Autodesk Inventor part; units mm, degrees
ref_plane "YZ Plane" through (0, 0, 0) normal (1, 0, 0) x (0, 1, 0)
ref_plane "XZ Plane" through (0, 0, 0) normal (0, 1, 0) x (-1, 0, 0)
ref_plane "XY Plane" through (0, 0, 0) normal (0, 0, 1) x (1, 0, 0)
sketch "Sketch1" plane through (0, 0, 0) normal (1, 0, 0) x (0, 1, 0)
  line L0 (44.6473, -162.2528) -> (44.6473, 101.2722)
  line L1 (-18.8527, 107.6222) -> (-3.6127, 107.6222)
  line L2 (-3.6127, 107.6222) -> (-3.6127, 101.2722)
  line L3 (-18.8527, 101.0377) -> (-18.8527, 107.6222)
  line L4 (2.7373, 107.6222) -> (17.9773, 107.6222)
  line L5 (17.9773, 107.6222) -> (17.9773, 101.2722)
  line L6 (2.7373, 101.2722) -> (2.7373, 107.6222)
  line L7 (24.3273, 107.6222) -> (39.5673, 107.6222)
  line L8 (39.5673, 107.6222) -> (39.5673, 101.2722)
  line L9 (24.3273, 101.2722) -> (24.3273, 107.6222)
  line L10 (39.5673, 101.2722) -> (44.6473, 101.2722)
  line L11 (24.3273, 101.2722) -> (17.9773, 101.2722)
  line L12 (2.7373, 101.2722) -> (-3.6127, 101.2722)
  line L13 (44.6473, -30.4903) -> (-18.8527, -30.4903) construction
  line L14 (-3.6127, -168.6028) -> (-3.6127, -162.2528)
  line L15 (17.9773, -168.6028) -> (17.9773, -162.2528)
  line L16 (2.7373, -162.2528) -> (2.7373, -168.6028)
  line L17 (39.5673, -168.6028) -> (39.5673, -162.2528)
  line L18 (24.3273, -162.2528) -> (24.3273, -168.6028)
  line L19 (39.5673, -162.2528) -> (44.6473, -162.2528)
  line L20 (24.3273, -162.2528) -> (17.9773, -162.2528)
  line L21 (2.7373, -162.2528) -> (-3.6127, -162.2528)
  line L22 (24.3273, -168.6028) -> (39.5673, -168.6028)
  line L23 (-18.8527, -168.6028) -> (-3.6127, -168.6028)
  line L24 (2.7373, -168.6028) -> (17.9773, -168.6028)
  line L25 (-3.6127, 107.6222) -> (-18.8527, 107.6222)
  line L26 (39.5673, 107.6222) -> (24.3273, 107.6222)
  line L27 (17.9773, 107.6222) -> (2.7373, 107.6222)
  line L28 (-18.8527, -20.9653) -> (-12.5027, -20.9653)
  line L29 (-12.5027, -20.9653) -> (-12.5027, 4.4347)
  line L30 (-12.5027, 4.4347) -> (-18.8527, 4.4347)
  line L31 (-18.8527, 23.4847) -> (-12.5027, 23.4847)
  line L32 (-12.5027, 23.4847) -> (-12.5027, 48.8847)
  line L33 (-12.5027, 48.8847) -> (-18.8527, 48.8847)
  line L34 (-18.8527, 67.9347) -> (-12.5027, 67.9347)
  line L35 (-12.5027, 67.9347) -> (-12.5027, 93.3347)
  line L36 (-12.5027, 93.3347) -> (-18.8527, 93.3347)
  line L37 (-3.6127, -168.6028) -> (-3.6127, -162.2528)
  line L38 (2.7373, -162.2528) -> (-3.6127, -162.2528)
  line L39 (-18.8527, -40.0153) -> (-12.5027, -40.0153)
  line L40 (-12.5027, -40.0153) -> (-12.5027, -65.4153)
  line L41 (-12.5027, -65.4153) -> (-18.8527, -65.4153)
  line L42 (-18.8527, -84.4653) -> (-12.5027, -84.4653)
  line L43 (-12.5027, -84.4653) -> (-12.5027, -109.8653)
  line L44 (-12.5027, -109.8653) -> (-18.8527, -109.8653)
  line L45 (-18.8527, -128.9153) -> (-12.5027, -128.9153)
  line L46 (-12.5027, -128.9153) -> (-12.5027, -154.3153)
  line L47 (-12.5027, -154.3153) -> (-18.8527, -154.3153)
  line L48 (-18.8527, 107.6222) -> (-18.8527, 93.3347)
  line L49 (-18.8527, 67.9347) -> (-18.8527, 48.8847)
  line L50 (-18.8527, 23.4847) -> (-18.8527, 4.4347)
  line L51 (-18.8527, -20.9653) -> (-18.8527, -40.0153)
  line L52 (-18.8527, -65.4153) -> (-18.8527, -84.4653)
  line L53 (-18.8527, -109.8653) -> (-18.8527, -128.9153)
  line L54 (-18.8527, -154.3153) -> (-18.8527, -168.6028)
  point P0 (0, 0)
  dimension "d2" = 15.24
  dimension "d3" = 6.35
  dimension "d4" = 15.24
  dimension "d5" = 6.35
  dimension "d7" = 15.24
  dimension "d8" = 9.525
  dimension "d9" = 19.05
  dimension "d10" = 19.05
  dimension "d12" = 25.4
  dimension "d13" = 25.4
  dimension "d14" = 25.4
  dimension "d16" = 6.35
  dimension "d17" = 6.35
  dimension "d20" = 276.225
extrude "Extrusion1" add sketch "Sketch1" along normal blind 6.35
equation "\"d10\" = d9"
equation "\"d13\" = d12"
equation "\"d14\" = d12"
properties part number "Front_Back" material "UHMW, White"
Part model, mm, in its own coordinate system. A direction names the side the tool comes from. Coordinates: 2 decimals unless noted, no trailing zeros. Write each loop counter-clockwise with the first axis right and the second up, starting at its lowest first coordinate (ties: lowest second). Pieces come first, ordered by that corner, then holes. Notation, with made-up numbers: (14.5, 59.25) - (34.5, 59.25) arc R18 cw to (34.5, 82.25) - close; hole circle Ø9 at (-13.5, 70). An arc over 180 degrees is marked (long way). Put each result on its own line as item: value.
1. Band-saw the part on A-A (y = -1). Write the cut outline in (x, z).
Final values:
outline: (0, -162.25) - (6.35, -162.25) - (6.35, 101.27) - (0, 101.27) - close
2. Probe line 1 along Z through (x, y) = (4.25, 22.5); line 2 along Y through (x, z) = (5.5, 0.5). List the from-to ranges inside material, lowest first. Write a range as [from, to].
Final values:
line 1: z = [-162.25, 101.27]
line 2: y = [-12.5, 44.65]
3. Flat gauge pins, fed straight in: pin 1 Ø2 at (x, z) = (5, 78.5) entering from -Y; pin 2 Ø3 at (x, z) = (4.5, -167) entering from +Y; pin 3 Ø1.5 at (x, y) = (3, 41.5) entering from +Z. Where does each tip first touch, or does it go through?
Final values:
pin 1: stops at y = -12.5
pin 2: stops at y = 39.57
pin 3: stops at z = 101.27
4. 3-axis set-ups, long thin cutter, end or side, ignore diameter. For faces 1 (the flat face through (3, -16, -84.465)), 2 (the flat face through (3, 21, -162.253)), 3 (the flat face through (3, 17.977, 104)), 4 (the flat face through (3, 42, 101.272)): which of +Z, -Z, +X, -X, +Y, -Y reach the whole face in a straight line?
Final values:
face 1: +X, -X, -Y
face 2: -Z, +X, -X
face 3: +Z, +X, -X
face 4: +Z, +X, -X, +Y
5. Two-plate mould, pull along Y, no slides. Class faces 5 (the flat face through (3, 2.737, -165)), 6 (the flat face through (3, 44.647, -32)), 7 (the flat face through (3, -12.503, -141)): +Y half, -Y half, draft (parallel to the pull), parting line (faces both ways), or undercut.
Final values:
face 5: undercut
face 6: +Y half
face 7: -Y half
6. Band-saw the part on B-B (z = 44). Write the cut outline in (x, y).
Final values:
outline: (0, -12.5) - (6.35, -12.5) - (6.35, 44.65) - (0, 44.65) - close
